Design review of the part built by this model. Coordinates are the model's own, in mm. Face numbers are marked on the shaded views. A direction names the side the tool comes from. Coordinates: 2 decimals unless noted, no trailing zeros. Write each loop counter-clockwise with the first axis right and the second up, starting at its lowest first coordinate (ties: lowest second). Pieces come first, ordered by that corner, then holes.
Q1. Add section D-D, the plane y = 10.5. Give the boundary of the cut face in (x, z) (3 decimals).
Q2. Add section B-B, the plane x = 0. Give the boundary of the cut face in (y, z) (3 decimals), plus the area to 3 significant figures.
Q3. Add section A-A, the plane z = 0. Give the boundary of the cut face in (x, y), plus the area to 3 significant figures.
Q4. To check wall thickness, follow probe 1 along Y at (x, z) = (2.5, -7); probe 2 along X at (y, z) = (45, 4.5); probe 3 along Z at (x, y) = (1.5, 17.5). State the ranges of each line that lie inside material, in increasing order.
Q5. Clearance check with flat-ended pins moving along their axes: pin 1 Ø1.5 at (x, y) = (1.5, 32.5) entering from -Z; pin 2 Ø4 at (x, y) = (3.5, 41) entering from +Z; pin 3 Ø1 at (x, z) = (5, 3.5) entering from +Y; pin 4 Ø5 at (x, z) = (3.5, -5) entering from +Y. State where each tip first meets the part, or that it passes through.
Q6. Machinability: for the marked faces 1, 2 and 3, which of the approach directions +Z, -Z, +X, -X, +Y, -Y give a long, thin tool a straight path to every point of the face, cutting with its end or side? Answer none if there is none.
Q7. Add section C-C, the plane y = 20. Give the boundary of the cut face in (x, z), plus the area to 3 significant figures.
from build123d import *

# Parameters (mm, degrees)
SKETCH2_W          = 2.25
SKETCH2_H          = 2.25
CUT_EXTRUDE1_DEPTH = 15
CHAMFER1_SIZE      = 0.5
CHAMFER2_SIZE      = 0.5


with BuildPart() as part:
    # Sketch1 → Revolve1 (revolve)
    with BuildSketch(Plane.XY, mode=Mode.PRIVATE) as revolve1_sk:
        Polygon((0, 0), (5, 0), (5, 15), (8, 15), (8, 18), (5, 18), (5, 85), (0, 85), align=None)
    revolve(revolve1_sk.sketch.rotate(Axis((0, 85, 0), (0, -1, 0)), 180), axis=Axis((0, 85, 0), (0, -1, 0)))

    # Sketch2 → Cut-Extrude1 (cut)
    with BuildSketch(Plane.XZ):
        with Locations((0, 5)):
            Rectangle(SKETCH2_W, SKETCH2_H)
    extrude(amount=-CUT_EXTRUDE1_DEPTH, mode=Mode.SUBTRACT)

    # Chamfer1
    chamfer1_edges = [part.edges().sort_by_distance(p)[0] for p in [
        (8, 18, 0),
        (8, 15, 0),
    ]]
    chamfer(chamfer1_edges, length=CHAMFER1_SIZE)

    # Chamfer2
    chamfer2_edges = [part.edges().sort_by_distance(p)[0] for p in [
        (0, 0, -5),
        (5, 85, 0),
    ]]
    chamfer(chamfer2_edges, length=CHAMFER2_SIZE)


solid = part.part
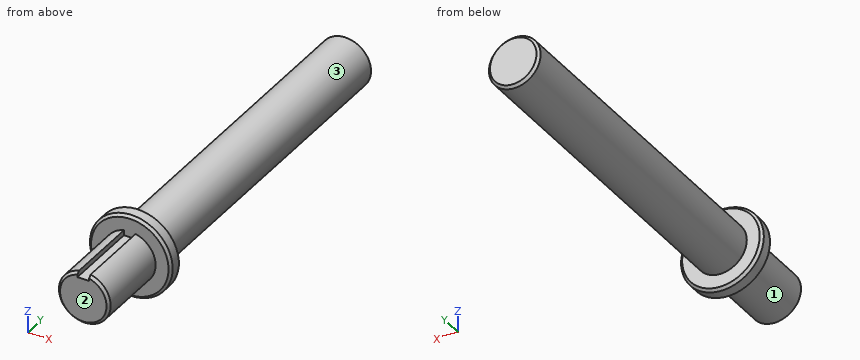
Here are the results:
1. outline: (-1.125, 3.875) - (-1.125, 4.872) arc R5 ccw (long way) to (1.125, 4.872) - (1.125, 3.875) - close
2. outline: (0, -4.5) - (0.5, -5) - (15, -5) - (15, -7.5) - (15.5, -8) - (17.5, -8) - (18, -7.5) - (18, -5) - (84.5, -5) - (85, -4.5) - (85, 4.5) - (84.5, 5) - (18, 5) - (18, 7.5) - (17.5, 8) - (15.5, 8) - (15, 7.5) - (15, 3.875) - (0, 3.875) - close
2. area: 850 mm2
3. outline: (-8, 15.5) - (-7.5, 15) - (-5, 15) - (-5, 0.5) - (-4.5, 0) - (4.5, 0) - (5, 0.5) - (5, 15) - (7.5, 15) - (8, 15.5) - (8, 17.5) - (7.5, 18) - (5, 18) - (5, 84.5) - (4.5, 85) - (-4.5, 85) - (-5, 84.5) - (-5, 18) - (-7.5, 18) - (-8, 17.5) - close
3. area: 867 mm2
4. probe 1: y = 15 to 18
4. probe 2: x = -2.18 to 2.18
4. probe 3: z = -7.86 to 7.86
5. pin 1: stops at z = -4.94
5. pin 2: stops at z = 4.77
5. pin 3: stops at y = 18
5. pin 4: stops at y = 85
6. face 1: -Y
6. face 2: +Z, -Z, +X, -X, -Y
6. face 3: +Y
7. outline: circle Ø10 at (0, 0)
7. area: 78.5 mm2
